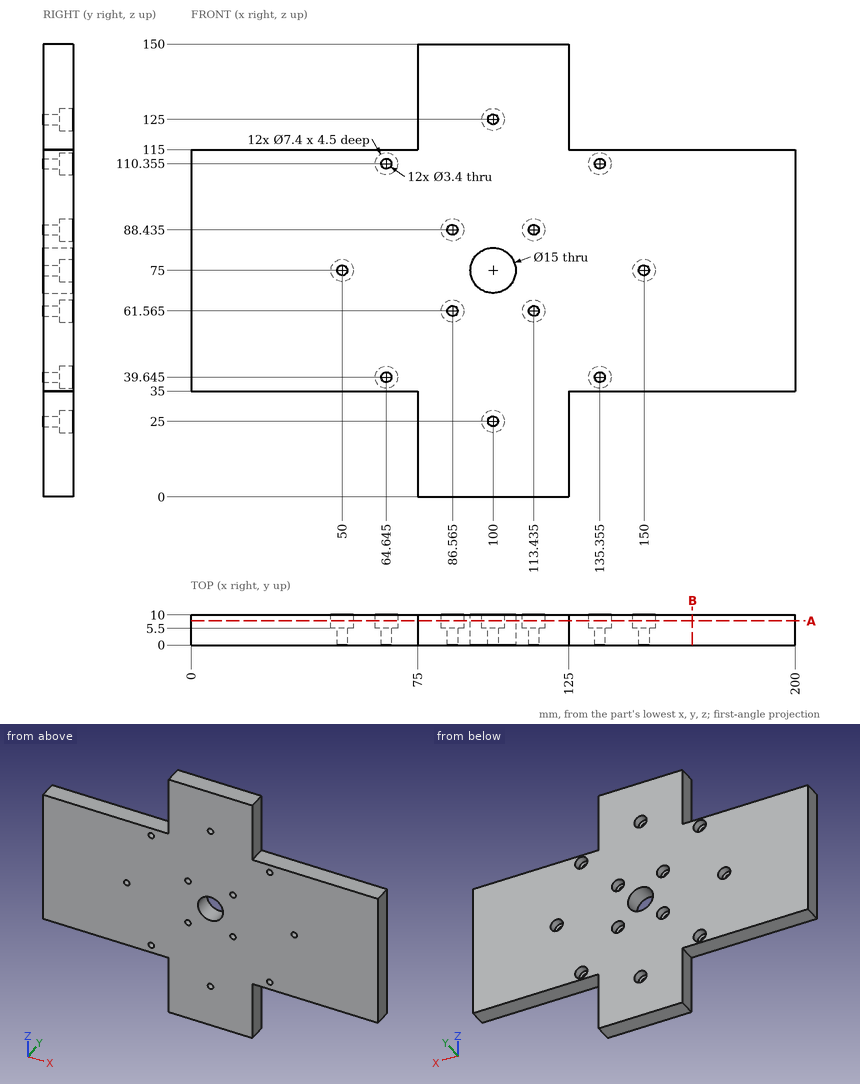
Part print with two shaded views. Sizes in mm from the minimum x, y, z corner. Round coordinates to 2 decimals unless told otherwise and drop trailing zeros. Loops run counter-clockwise (first coordinate to the right, second up) from the corner with the lowest first, then second, coordinate; pieces in that order, holes last. Notation, with made-up numbers: (65.5, 22) - (76.5, 22) arc R22 cw to (76.5, 47) - close; hole circle Ø1 at (36.25, 88.5). An arc over 180 degrees is marked (long way). Answer as a JSON object with one key per item and string values.
Item 1: Band-saw the part on A-A on y = 8. State how many separate pieces and enclosed holes the cut face has, plus the area to 3 significant figures.
Output:
{"separate pieces": "1", "enclosed holes": "13", "area": "18,800 mm2"}
Item 2: Pin check, flat tips, straight feed: pin 1 (1 mm diameter, centred on x = 73.5, y = 7.5, fed in from +Z); pin 2 (5 mm diameter, centred on y = 6, z = 136.5, fed in from +X); pin 3 (2 mm diameter, centred on x = 113.44, z = 61.56, fed in from -Y); pin 4 (6 mm diameter, centred on x = 86.56, z = 61.56, fed in from +Y). Stop position of each tip, or through.
Output:
{"pin 1": "z = 115", "pin 2": "x = 125", "pin 3": "through", "pin 4": "y = 5.5"}
Item 3: Wall check: L1, parallel to X at y = 3, z = 40; L2, parallel to X at y = 2.4, z = 75; L3, parallel to X at y = 6.7, z = 75. Give the ranges that are in metal, low to high.
Output:
{"L1": "0 to 62.98, 66.31 to 133.69, 137.02 to 200", "L2": "0 to 48.3, 51.7 to 92.5, 107.5 to 148.3, 151.7 to 200", "L3": "0 to 46.3, 53.7 to 92.5, 107.5 to 146.3, 153.7 to 200"}
Item 4: Band-saw the part on B-B on x = 166. List the corners of the cut face in (y, z), plus the area to 3 significant figures.
Output:
{"outline": "(0, 35) - (10, 35) - (10, 115) - (0, 115) - close", "area": "800 mm2"}
